Source: CAD feature listing. Evaluate the final solid. Frame: model axes, mm. A direction names the side the tool comes from. Give positions to 0.01 mm unless a question says otherwise; leave off trailing zeros. Order: outer loops, then holes, each group sorted by start corner. A loop starts at its lowest first (then second) coordinate and runs counter-clockwise, first axis right, second up. Notation, with made-up numbers: M 79,79.25 L 119,79.25 A12 cw 119,96.25 Z; hole C 38.25,57 d9. An arc over 180 degrees is marked long. Use CSV: the item, a comma, the result in double quotes. Start each with the question number.
1. Mould query, pull axis X, two halves, no side actions, for faces 1 (the flat face through (25, 1.75, -6)), 2 (the flat face through (56, 6, -9)), 3 (the cylindrical face through (52.451, 2.035, -7.449)). Classes: released by +X, released by -X, zero draft, split by the parting line, or undercut.
2. Section query A-A, the plane z = -2.75. Return the cut outline in (x, y) (3 decimals), plus the area to 3 significant figures.
3. Line query: line 1 along Y through (x, z) = (-3, -11.6) (3 decimals); line 2 along X through (y, z) = (1.4, -2.75) (3 decimals); line 3 along X through (y, z) = (5.75, -8.45) (3 decimals). Output: solid intervals per line, ascending. Write a range as [from, to].
4. Section query C-C, the plane y = 5.75. Return the cut outline in (x, z) (3 decimals).
5. Reachability of faces 4 (the flat face through (-3, 10, -7.75)), 5 (the flat face through (25, 0, -6)), 6 (the flat face through (0, 10, -10)) from +Z, -Z, +X, -X, +Y, -Y: full face, straight path, thin tool, end or side. Return the list, or none.
6. Section query B-B, the plane x = -3. Return the cut outline in (y, z) (3 decimals).
7. Section query D-D, the plane z = -9.5. Return the cut outline in (x, y) (3 decimals), plus the area to 3 significant figures.
8. Pin query (flat end, axial travel): P1, Ø3, axis at x = 52, y = 13, coming from the +Z side; P2, Ø4, axis at x = 24.5, z = -8, coming from the +Y side. Return the tip coordinate at first contact, or that it passes through.
from build123d import *

# Parameters (mm, degrees)
SKETCH1_W                  = 50
SKETCH1_H                  = 12.5
BASE_DEPTH                 = 1.75
SKETCH2_R                  = 1.375
CHASSISMOUNTINGHOLES_DEPTH = 1.75
SKETCH3_W                  = 6
SKETCH3_H                  = 16.75
SKETCH3_R                  = 1.375
BOSS_EXTRUDE2_DEPTH        = 1.75
BOSS_EXTRUDE3_DEPTH        = 1.75
SKETCH5_W                  = 6
SKETCH5_H                  = 15
SKETCH5_R                  = 1.375
BOSS_EXTRUDE4_DEPTH        = 3
BOSS_EXTRUDE5_DEPTH        = 1.75
FILLET1_R                  = 1


with BuildPart() as part:
    # Sketch1 → base (new body)
    with BuildSketch(Plane(origin=(0, 0, 0), x_dir=(1, 0, 0), z_dir=(0, 1, 0))):
        with Locations((25, 6.25)):
            Rectangle(SKETCH1_W, SKETCH1_H)
    extrude(amount=BASE_DEPTH)

    # Sketch2 → chassisMountingHoles (cut)
    with BuildSketch(Plane(origin=(0, 1.75, 0), x_dir=(1, 0, 0), z_dir=(0, 1, 0))):
        with Locations(Location((3, 2.75, 0), (0, 0, 270))):
            Circle(SKETCH2_R)
        with Locations(Location((47, 2.75, 0), (0, 0, 90))):
            Circle(SKETCH2_R)
    extrude(amount=-CHASSISMOUNTINGHOLES_DEPTH, mode=Mode.SUBTRACT)

    # Sketch3 → Boss-Extrude2 (add)
    with BuildSketch(Plane(origin=(0, 0, -12.5), x_dir=(-1, 0, 0), z_dir=(0, 0, -1))):
        with Locations((3, 8.375)):
            Rectangle(SKETCH3_W, SKETCH3_H)
        with Locations((3, 12.75)):
            Circle(SKETCH3_R, mode=Mode.SUBTRACT)
        with Locations((3, 5.75)):
            Circle(SKETCH3_R, mode=Mode.SUBTRACT)
        with Locations((-53, 8.375)):
            Rectangle(SKETCH3_W, SKETCH3_H)
        with Locations(Location((-53, 12.75, 0), (0, 0, 180))):
            Circle(SKETCH3_R, mode=Mode.SUBTRACT)
        with Locations(Location((-53, 5.75, 0), (0, 0, 180))):
            Circle(SKETCH3_R, mode=Mode.SUBTRACT)
    extrude(amount=-BOSS_EXTRUDE2_DEPTH)

    # Sketch4 → Boss-Extrude3 (add)
    with BuildSketch(Plane(origin=(0, 1.75, 0), x_dir=(1, 0, 0), z_dir=(0, 1, 0))):
        Polygon((50, 0), (56, 10.75), (50, 10.75), align=None)
        Polygon((-6, 10.75), (0, 10.75), (0, 0), align=None)
    extrude(amount=-BOSS_EXTRUDE3_DEPTH)

    # Sketch5 → Boss-Extrude4 (add)
    with BuildSketch(Plane.XY.offset(-10.75)):
        with Locations((-3, 9.25)):
            Rectangle(SKETCH5_W, SKETCH5_H)
        with Locations(Location((-3, 5.75, 0), (0, 0, 180))):
            Circle(SKETCH5_R, mode=Mode.SUBTRACT)
        with Locations(Location((-3, 12.75, 0), (0, 0, 180))):
            Circle(SKETCH5_R, mode=Mode.SUBTRACT)
        with Locations((53, 9.25)):
            Rectangle(SKETCH5_W, SKETCH5_H)
        with Locations((53, 5.75)):
            Circle(SKETCH5_R, mode=Mode.SUBTRACT)
        with Locations((53, 12.75)):
            Circle(SKETCH5_R, mode=Mode.SUBTRACT)
    extrude(amount=BOSS_EXTRUDE4_DEPTH)

    # Sketch6 → Boss-Extrude5 (add)
    with BuildSketch(Plane.XZ):
        Polygon((-6, -10.75), (-6, 0), (0, 0), align=None)
        Polygon((56, 0), (50, 0), (56, -10.75), align=None)
    extrude(amount=-BOSS_EXTRUDE5_DEPTH)

    # Fillet1
    fillet1_edges = [part.edges().sort_by_distance(p)[0] for p in [
        (53, 1.75, -7.75),
        (50, 1.75, -10.125),
        (0, 1.75, -10.125),
        (-3, 1.75, -7.75),
    ]]
    fillet(fillet1_edges, radius=FILLET1_R)


solid = part.part
Result set:
1,face 1,"undercut"
1,face 2,"released by +X"
1,face 3,"zero draft"
2,outline,"M -6,0 L 1.625,0 L 1.625,1.75 L -6,1.75 Z; M 4.375,0 L 45.625,0 L 45.625,1.75 L 4.375,1.75 Z; M 48.375,0 L 56,0 L 56,1.75 L 48.375,1.75 Z"
2,area,"98.9 mm2"
3,line 1,"[0, 4.375], [7.125, 11.375], [14.125, 16.75]"
3,line 2,"[-6, 1.625], [4.375, 45.625], [48.375, 56]"
3,line 3,"[-6, -4.375], [-1.625, 0], [50, 51.625], [54.375, 56]"
4,outline,"M -6,-12.5 L -4.375,-12.5 L -4.375,-7.75 L -6,-7.75 Z; M -1.625,-12.5 L 0,-12.5 L 0,-7.75 L -1.625,-7.75 Z; M 50,-12.5 L 51.625,-12.5 L 51.625,-7.75 L 50,-7.75 Z; M 54.375,-12.5 L 56,-12.5 L 56,-7.75 L 54.375,-7.75 Z"
5,face 4,"+Z, +X, -X, +Y"
5,face 5,"+Z, -Z, +X, -X, -Y"
5,face 6,"+Z, -Z, +Y"
6,outline,"M 0,-12.5 L 4.375,-12.5 L 4.375,-7.75 L 2.75,-7.75 A1 cw 1.75,-6.75 L 1.75,0 L 0,0 Z; M 7.125,-12.5 L 11.375,-12.5 L 11.375,-7.75 L 7.125,-7.75 Z; M 14.125,-12.5 L 16.75,-12.5 L 16.75,-7.75 L 14.125,-7.75 Z"
7,outline,"M -6,0 L 56,0 L 56,16.75 L 50,16.75 L 50,2.75 A1 cw 49,1.75 L 1,1.75 A1 cw 0,2.75 L 0,16.75 L -6,16.75 Z; hole C -3,5.75 d2.75; hole C -3,12.75 d2.75; hole C 53,5.75 d2.75; hole C 53,12.75 d2.75"
7,area,"265 mm2"
8,P1,"z = -7.75"
8,P2,"y = 1.75"
